from build123d import *

# Parameters (mm, degrees)
SKETCH4_W                  = 21.59
SKETCH4_H                  = 21.59
SKETCH4_W_2                = 19.05
SKETCH4_H_2                = 19.05
BOSS_EXTRUDE2_DEPTH        = 161.925
FILLET1_R                  = 2.54
F_10_CLEARANCE_HOLE1_D     = 5.1054
F_10_CLEARANCE_HOLE1_DEPTH = 12.7
F_10_CLEARANCE_HOLE1_TIP   = 1.533816902
F_10_CLEARANCE_HOLE2_D     = 5.1054
F_10_CLEARANCE_HOLE2_DEPTH = 12.7
F_10_CLEARANCE_HOLE2_TIP   = 1.533816902


with BuildPart() as part:
    # Sketch4 → Boss-Extrude2 (new body)
    with BuildSketch(Plane.XY):
        Rectangle(SKETCH4_W, SKETCH4_H)
        Rectangle(SKETCH4_W_2, SKETCH4_H_2, mode=Mode.SUBTRACT)
    extrude(amount=BOSS_EXTRUDE2_DEPTH)

    # Fillet1
    fillet1_edges = [part.edges().sort_by_distance(p)[0] for p in [
        (-9.525, 9.525, 80.9625),
        (-9.525, -9.525, 80.9625),
        (9.525, -9.525, 80.9625),
        (9.525, 9.525, 80.9625),
        (-10.795, 10.795, 80.9625),
        (10.795, 10.795, 80.9625),
        (10.795, -10.795, 80.9625),
        (-10.795, -10.795, 80.9625),
    ]]
    fillet(fillet1_edges, radius=FILLET1_R)

    # #10 Clearance Hole1
    with Locations(Plane(origin=(0, 10.795, 0), x_dir=(1, 0, 0), z_dir=(0, 1, 0))):
        with Locations((0, -12.7)):
            Hole(F_10_CLEARANCE_HOLE1_D / 2, depth=F_10_CLEARANCE_HOLE1_DEPTH)
            with Locations((0, 0, -(F_10_CLEARANCE_HOLE1_DEPTH + F_10_CLEARANCE_HOLE1_TIP / 2))):  # 118° drill point
                Cone(0, F_10_CLEARANCE_HOLE1_D / 2, F_10_CLEARANCE_HOLE1_TIP, mode=Mode.SUBTRACT)

    # #10 Clearance Hole2
    with Locations(Plane.ZY.offset(10.795)):
        with Locations((149.225, 0)):
            Hole(F_10_CLEARANCE_HOLE2_D / 2, depth=F_10_CLEARANCE_HOLE2_DEPTH)
            with Locations((0, 0, -(F_10_CLEARANCE_HOLE2_DEPTH + F_10_CLEARANCE_HOLE2_TIP / 2))):  # 118° drill point
                Cone(0, F_10_CLEARANCE_HOLE2_D / 2, F_10_CLEARANCE_HOLE2_TIP, mode=Mode.SUBTRACT)


solid = part.part
Source: CAD feature listing. Evaluate the final solid. Frame: model axes, mm. A direction names the side the tool comes from. Round coordinates to 2 decimals unless told otherwise and drop trailing zeros. Order: outer loops, then holes, each group sorted by start corner. A loop starts at its lowest first (then second) coordinate and runs counter-clockwise, first axis right, second up. Notation, with made-up numbers: (71.5, -29.75) - (75.5, -29.75) arc R18 cw to (75.5, -17.75) - close; hole circle Ø6 at (88, 7). An arc over 180 degrees is marked (long way). Use a Markdown table: item, result. Add a question column.
1. Line query: probe 1 along X at (y, z) = (-4, 126) (3 decimals); probe 2 along Z at (x, y) = (0, 9.9) (3 decimals). Output: solid intervals per line, ascending.
2. Set-up query: faces 1 (the flat face through (0, -9.525, 80)), 2 (the cylindrical face through (-10.151, 0.112, 151.775)), 3 (the flat face through (-10.795, 0, 80)). Return all of +Z, -Z, +X, -X, +Y, -Y with unobstructed straight access to the full face (end or side cutting, diameter ignored); none if empty.
3. Section query B-B (x = 0). Return the cut outline in (y, z) (3 decimals).
4. Section query D-D (z = 12.7). Return the cut outline in (x, y) (3 decimals).
5. Section query A-A (y = -4). Return the cut outline in (x, z) (3 decimals), then the cut area to 3 significant figures.
6. First-contact query: pin 1 (3 mm diameter, centred on x = 0, z = 12.7, fed in from +Y) (3 decimals); pin 2 (1 mm diameter, centred on x = 7.5, y = 8.5, fed in from +Z). Flat tips, straight axial feed; report the tip coordinate or a pass-through.
7. Section query C-C (z = 64.5). Return the cut outline in (x, y) (3 decimals).
8. Mould query, pull axis Z, two halves, no side actions, for faces 4 (the flat face through (1, -10, 161.925)), 5 (the cylindrical face through (8.76, -8.8, 82.1)), 6 (the cylindrical face through (0.553, 10.151, 15.192)). Classes: +Z half, -Z half, draft (parallel to the pull), parting line (faces both ways), or undercut.
Derived:
| question | item | result |
|---|---|---|
| 1 | probe 1 | -10.795 to -9.525, 9.525 to 10.795 |
| 1 | probe 2 | 0 to 10.147, 15.253 to 161.925 |
| 2 | face 1 | +Z, -Z |
| 2 | face 2 | -X |
| 2 | face 3 | +Z, -Z, -X, +Y, -Y |
| 3 | outline | (-10.795, 0) - (-9.525, 0) - (-9.525, 161.925) - (-10.795, 161.925) - close; (9.525, 0) - (10.795, 0) - (10.795, 10.147) - (9.525, 10.147) - close; (9.525, 15.253) - (10.795, 15.253) - (10.795, 161.925) - (9.525, 161.925) - close |
| 4 | outline | (-10.795, -8.255) arc R2.54 ccw to (-8.255, -10.795) - (8.255, -10.795) arc R2.54 ccw to (10.795, -8.255) - (10.795, 8.255) arc R2.54 ccw to (8.255, 10.795) - (2.553, 10.795) - (2.553, 9.525) - (6.985, 9.525) arc R2.54 cw to (9.525, 6.985) - (9.525, -6.985) arc R2.54 cw to (6.985, -9.525) - (-6.985, -9.525) arc R2.54 cw to (-9.525, -6.985) - (-9.525, 6.985) arc R2.54 cw to (-6.985, 9.525) - (-2.553, 9.525) - (-2.553, 10.795) - (-8.255, 10.795) arc R2.54 ccw to (-10.795, 8.255) - close |
| 5 | outline | (-10.795, 0) - (-9.525, 0) - (-9.525, 161.925) - (-10.795, 161.925) - close; (9.525, 0) - (10.795, 0) - (10.795, 161.925) - (9.525, 161.925) - close |
| 5 | area | 411 mm2 |
| 6 | pin 1 | y = -9.525 |
| 6 | pin 2 | through |
| 7 | outline | (-10.795, -8.255) arc R2.54 ccw to (-8.255, -10.795) - (8.255, -10.795) arc R2.54 ccw to (10.795, -8.255) - (10.795, 8.255) arc R2.54 ccw to (8.255, 10.795) - (-8.255, 10.795) arc R2.54 ccw to (-10.795, 8.255) - close; hole (-9.525, -6.985) arc R2.54 ccw to (-6.985, -9.525) - (6.985, -9.525) arc R2.54 ccw to (9.525, -6.985) - (9.525, 6.985) arc R2.54 ccw to (6.985, 9.525) - (-6.985, 9.525) arc R2.54 ccw to (-9.525, 6.985) - close |
| 8 | face 4 | +Z half |
| 8 | face 5 | draft |
| 8 | face 6 | undercut |
